Read the model definition and answer for the solid it produces. Units are mm, in the model's axes. Round coordinates to 2 decimals unless told otherwise and drop trailing zeros. Order: outer loops, then holes, each group sorted by start corner. A loop starts at its lowest first (then second) coordinate and runs counter-clockwise, first axis right, second up.
from build123d import *

# Parameters (mm, degrees)
AUFSATZ_LINEAR_AUSTRAGEN1_DEPTH = 1.5
SCHNITT_LINEAR_AUSTRAGEN3_DEPTH = 25.287033578
SKIZZE8_R                       = 1.2
SCHNITT_LINEAR_AUSTRAGEN4_DEPTH = 25.287033578


with BuildPart() as part:
    # Skizze1 → Aufsatz-Linear austragen1 (new body)
    with BuildSketch(Plane.XY):
        with BuildLine():
            Line((15.5, -14.4), (-15.5, -14.4))
            ThreePointArc((-15.5, -14.4), (-18.328427125, -13.228427125), (-19.5, -10.4))
            Line((-19.5, -10.4), (-19.5, 10.4))
            ThreePointArc((-19.5, 10.4), (-18.328427125, 13.228427125), (-15.5, 14.4))
            Line((-15.5, 14.4), (15.5, 14.4))
            ThreePointArc((15.5, 14.4), (18.328427125, 13.228427125), (19.5, 10.4))
            Line((19.5, 10.4), (19.5, -10.4))
            ThreePointArc((19.5, -10.4), (18.328427125, -13.228427125), (15.5, -14.4))
        make_face()
    extrude(amount=AUFSATZ_LINEAR_AUSTRAGEN1_DEPTH)

    # Skizze2 → Schnitt-Linear austragen3 (cut, through all)
    with BuildSketch(Plane.XY.offset(1.5)):
        with BuildLine():
            Line((15.5, 11.3), (-9.786857257, 11.3))
            ThreePointArc((-9.786857257, 11.3), (-11.832490505, 10.737351395), (-13.302637407, 9.207692308))
            ThreePointArc((-13.302637407, 9.207692308), (-13.732233047, 8.632233047), (-14.307692308, 8.202637407))
            ThreePointArc((-14.307692308, 8.202637407), (-15.837351395, 6.732490505), (-16.4, 4.686857257))
            Line((-16.4, 4.686857257), (-16.4, -10.4))
            ThreePointArc((-16.4, -10.4), (-16.136396103, -11.036396103), (-15.5, -11.3))
            Line((-15.5, -11.3), (9.786857257, -11.3))
            ThreePointArc((9.786857257, -11.3), (11.832490505, -10.737351395), (13.302637407, -9.207692308))
            ThreePointArc((13.302637407, -9.207692308), (13.732233047, -8.632233047), (14.307692308, -8.202637407))
            ThreePointArc((14.307692308, -8.202637407), (15.837351395, -6.732490505), (16.4, -4.686857257))
            Line((16.4, -4.686857257), (16.4, 10.4))
            ThreePointArc((16.4, 10.4), (16.136396103, 11.036396103), (15.5, 11.3))
        make_face()
    extrude(amount=-SCHNITT_LINEAR_AUSTRAGEN3_DEPTH, mode=Mode.SUBTRACT)

    # Skizze8 → Schnitt-Linear austragen4 (cut, through all)
    with BuildSketch(Plane.XY.offset(1.5)):
        with Locations((-15.3, 10.2)):
            Circle(SKIZZE8_R)
        with Locations((15.3, -10.2)):
            Circle(SKIZZE8_R)
    extrude(amount=-SCHNITT_LINEAR_AUSTRAGEN4_DEPTH, mode=Mode.SUBTRACT)


solid = part.part
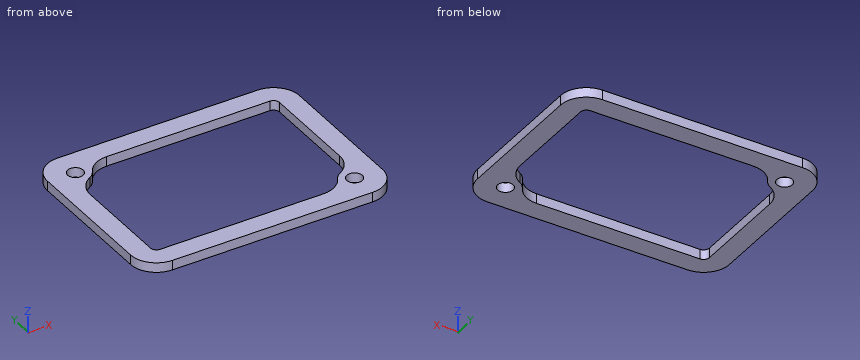
Q1. Straight lines are drawn through the part: probe 1 along Y at (x, z) = (15.3, 1.2); probe 2 along Y at (x, z) = (-15.3, 0.65); probe 3 along Y at (x, z) = (3, 0.4). For each, find the intervals that lie inside material, in ascending order.
Outcome:
probe 1: y = -14.4 to -11.4, -9 to -7.44, 11.3 to 14.4
probe 2: y = -14.4 to -11.3, 7.44 to 9, 11.4 to 14.4
probe 3: y = -14.4 to -11.3, 11.3 to 14.4
Q2. A cutting plane is placed at A-A, the plane y = 0.75. Give the vertices of the cut face in (x, z).
Outcome:
outline: (-19.5, 0) - (-16.4, 0) - (-16.4, 1.5) - (-19.5, 1.5) - close; (16.4, 0) - (19.5, 0) - (19.5, 1.5) - (16.4, 1.5) - close
Q3. A cutting plane is placed at B-B, the plane x = -4.5. Give the vertices of the cut face in (y, z).
Outcome:
outline: (-14.4, 0) - (-11.3, 0) - (-11.3, 1.5) - (-14.4, 1.5) - close; (11.3, 0) - (14.4, 0) - (14.4, 1.5) - (11.3, 1.5) - close
Q4. A cutting plane is placed at C-C, the plane z = 0.55. Give the vertices of the cut face in (x, y), plus the area to 3 significant figures.
Outcome:
outline: (-19.5, -10.4) arc R4 ccw to (-15.5, -14.4) - (15.5, -14.4) arc R4 ccw to (19.5, -10.4) - (19.5, 10.4) arc R4 ccw to (15.5, 14.4) - (-15.5, 14.4) arc R4 ccw to (-19.5, 10.4) - close; hole circle Ø2.4 at (-15.3, 10.2); hole (-16.4, -10.4) arc R0.9 ccw to (-15.5, -11.3) - (9.79, -11.3) arc R4 ccw to (13.3, -9.21) arc R2.5 cw to (14.31, -8.2) arc R4 ccw to (16.4, -4.69) - (16.4, 10.4) arc R0.9 ccw to (15.5, 11.3) - (-9.79, 11.3) arc R4 ccw to (-13.3, 9.21) arc R2.5 cw to (-14.31, 8.2) arc R4 ccw to (-16.4, 4.69) - close; hole circle Ø2.4 at (15.3, -10.2)
area: 386 mm2
